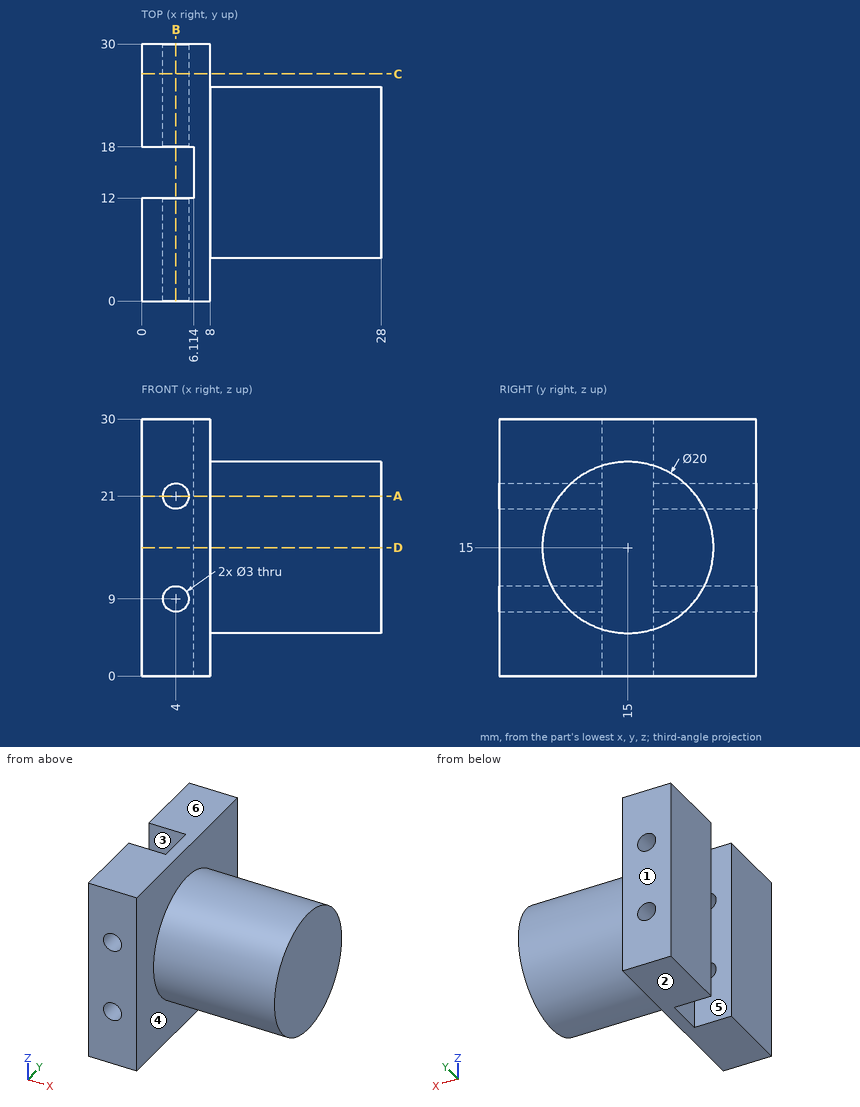
Here's the drawing with two shaded views (mm, measured from the low corner). I have some questions. A direction names the side the tool comes from. Round coordinates to 2 decimals unless told otherwise and drop trailing zeros. Write each loop counter-clockwise with the first axis right and the second up, starting at its lowest first coordinate (ties: lowest second). Pieces come first, ordered by that corner, then holes. Notation, with made-up numbers: M 34.5,71.5 L 93.5,71.5 A26 cw 93.5,105.5 Z; hole C 43,18.5 d4. An arc over 180 degrees is marked long. Answer in a Markdown table with one row per item. Add a question column.
Q1. Imagine slicing it at B-B (x = 4). Please give me the cut outline in (y, z).
Q2. On a 3-axis mill with a long thin cutter (end or side, diameter ignored), from which of +Z, -Z, +X, -X, +Y, -Y can I reach the whole of each face in a straight line? I mean the marked faces 4, 5 and 6. Say none if no direction works.
Q3. Imagine slicing it at D-D (z = 15). Please give me the cut outline in (x, y).
Q4. Imagine slicing it at C-C (y = 26.5). Please give me the cut outline in (x, z).
Q5. If I drill on line 1 (Z direction, x = 4.25, y = 20); line 2 (Y direction, x = 5.75, z = 15.25); line 3 (X direction, y = 4.75, z = 9), over which ranges is the centre line in solid material (lowest first)? Write a range as from..to.
Q6. If we mould it in two halves opening along Y, with no side actions, what happens to the marked faces 1, 2 and 3? For each: +Y half, -Y half, draft (parallel to the pull), parting line (faces both ways), or undercut.
Q7. Will these pins go through, and if not, where does the flat tip stop? pin 1 Ø2.5 at (x, z) = (4, 21) entering from +Y; pin 2 Ø2 at (x, z) = (16.5, 9.5) entering from -Y; pin 3 Ø12 at (x, z) = (18, 25.5) entering from +Y; pin 4 Ø10 at (x, z) = (14.5, 21) entering from +Y.
Q8. Imagine slicing it at A-A (z = 21). Please give me the cut outline in (x, y).
Values:
| question | item | result |
|---|---|---|
| 1 | outline | M 0,0 L 12,0 L 12,7.5 L 0,7.5 Z; M 0,10.5 L 12,10.5 L 12,19.5 L 0,19.5 Z; M 0,22.5 L 12,22.5 L 12,30 L 0,30 Z; M 18,0 L 30,0 L 30,7.5 L 18,7.5 Z; M 18,10.5 L 30,10.5 L 30,19.5 L 18,19.5 Z; M 18,22.5 L 30,22.5 L 30,30 L 18,30 Z |
| 2 | face 4 | +X |
| 2 | face 5 | +Z, -Z, -X |
| 2 | face 6 | +Z, +X, -X, +Y, -Y |
| 3 | outline | M 0,0 L 8,0 L 8,5 L 28,5 L 28,25 L 8,25 L 8,30 L 0,30 L 0,18 L 6.11,18 L 6.11,12 L 0,12 Z |
| 4 | outline | M 0,0 L 8,0 L 8,30 L 0,30 Z; hole C 4,9 d3; hole C 4,21 d3 |
| 5 | line 1 | 0..7.52, 10.48..19.52, 22.48..30 |
| 5 | line 2 | 0..12, 18..30 |
| 5 | line 3 | 0..2.5, 5.5..8 |
| 6 | face 1 | +Y half |
| 6 | face 2 | draft |
| 6 | face 3 | undercut |
| 7 | pin 1 | through |
| 7 | pin 2 | y = 6.07 |
| 7 | pin 3 | y = 23.93 |
| 7 | pin 4 | y = 24.95 |
| 8 | outline | M 0,0 L 2.5,0 L 2.5,12 L 0,12 Z; M 0,18 L 2.5,18 L 2.5,30 L 0,30 Z; M 5.5,0 L 8,0 L 8,7 L 28,7 L 28,23 L 8,23 L 8,30 L 5.5,30 L 5.5,18 L 6.11,18 L 6.11,12 L 5.5,12 Z |
